The listing builds one solid part. Answer for the finished solid, in the listing's coordinates (mm). A direction names the side the tool comes from. Round coordinates to 2 decimals unless told otherwise and drop trailing zeros. Order: outer loops, then holes, each group sorted by start corner. A loop starts at its lowest first (then second) coordinate and runs counter-clockwise, first axis right, second up. Notation, with made-up numbers: (-2, 62.5) - (12, 62.5) arc R20 cw to (12, 90.5) - close; hole circle Ø7 at (57, 50). An arc over 180 degrees is marked (long way). Write item = value, one per line.
from build123d import *

# Parameters (mm, degrees)
SKETCH1_R                      = 27.505813168
SKETCH1_R_2                    = 25.505813168
BOSS_EXTRUDE1_DEPTH            = 30
SKETCH2_R                      = 27.505813168
SKETCH2_R_2                    = 25.505813168
BOSS_EXTRUDE4_DEPTH            = 6
SKETCH2_4_R                    = 25.505813168
SKETCH2_4_R_2                  = 10.5
BOSS_EXTRUDE5_DEPTH            = 4
SKETCH2_5_R                    = 10.5
BOSS_EXTRUDE6_DEPTH            = 2
SKETCH3_R                      = 27.505813168
SKETCH3_R_2                    = 25.505813168
SKETCH3_R_3                    = 21.505813168
SKETCH3_W                      = 4
SKETCH3_H                      = 13
BOSS_EXTRUDE8_DEPTH            = 6
CUT_EXTRUDE3_REACH             = 53.664
CUT_EXTRUDE4_REACH             = 55.001
SKETCH9_R                      = 1
CUT_EXTRUDE4_DIRECTION_2_DEPTH = 54.001316173
FILLET9_R                      = 10
FILLET10_R                     = 1


# Some blends are built 0.0001 mm under size
with BuildPart() as part:
    # Sketch1 → Boss-Extrude1 (new body)
    with BuildSketch(Plane.YZ):
        with Locations(Location((0, 0, 0), (0, 0, 270))):
            Circle(SKETCH1_R)
        with Locations(Location((0, 0, 0), (0, 0, 270))):
            Circle(SKETCH1_R_2, mode=Mode.SUBTRACT)
    extrude(amount=BOSS_EXTRUDE1_DEPTH)

    # Sketch2 → Boss-Extrude4 (add)
    with BuildSketch(Plane.YZ.offset(30)):
        with Locations(Location((0, 0, 0), (0, 0, 270))):
            Circle(SKETCH2_R)
        with Locations(Location((0, 0, 0), (0, 0, 270))):
            Circle(SKETCH2_R_2, mode=Mode.SUBTRACT)
    extrude(amount=BOSS_EXTRUDE4_DEPTH)

    # Sketch2<4> → Boss-Extrude5 (add)
    with BuildSketch(Plane.YZ.offset(30)):
        with Locations(Location((0, 0, 0), (0, 0, 270))):
            Circle(SKETCH2_4_R)
        with Locations(Location((0, 0, 0), (0, 0, 270))):
            Circle(SKETCH2_4_R_2, mode=Mode.SUBTRACT)
    extrude(amount=BOSS_EXTRUDE5_DEPTH)

    # Sketch2<5> → Boss-Extrude6 (add)
    with BuildSketch(Plane.YZ.offset(30)):
        with Locations(Location((0, 0, 0), (0, 0, 270))):
            Circle(SKETCH2_5_R)
    extrude(amount=BOSS_EXTRUDE6_DEPTH)

    # Sketch3 → Boss-Extrude8 (add)
    # profile 1 of 6: a face of its own
    with BuildSketch(Plane(origin=(0, 0, 0), x_dir=(0, -1, 0), z_dir=(-1, 0, 0))):
        with Locations(Location((0, 0, 0), (0, 0, 270))):
            Circle(SKETCH3_R)
        with Locations(Location((0, 0, 0), (0, 0, 270))):
            Circle(SKETCH3_R_2, mode=Mode.SUBTRACT)
    # profile 2 of 6: a face of its own
    with BuildSketch(Plane(origin=(0, 0, 0), x_dir=(0, -1, 0), z_dir=(-1, 0, 0))):
        with Locations(Location((0, 0, 0), (0, 0, 270))):
            Circle(SKETCH3_R_2)
        Circle(SKETCH3_R_3, mode=Mode.SUBTRACT)
    # profile 3 of 6: a face of its own
    with BuildSketch(Plane(origin=(0, 0, 0), x_dir=(0, -1, 0), z_dir=(-1, 0, 0))):
        with BuildLine():
            ThreePointArc((12.5, 0), (3.375390485, 12.035644523), (-10.677078252, 6.5))
            Line((-10.677078252, 6.5), (0, 6.5))
            Line((0, 6.5), (7.5, 6.5))
            Line((7.5, 6.5), (7.5, -6.5))
            Line((7.5, -6.5), (0, -6.5))
            Line((0, -6.5), (-10.677078252, -6.5))
            ThreePointArc((-10.677078252, -6.5), (3.375390485, -12.035644523), (12.5, 0))
        make_face()
    # profile 4 of 6: a face of its own
    with BuildSketch(Plane(origin=(0, 0, 0), x_dir=(0, -1, 0), z_dir=(-1, 0, 0))):
        with BuildLine():
            Line((-20.5, -6.5), (-20.5, 6.5))
            ThreePointArc((-20.5, 6.5), (-21.505813168, 0), (-20.5, -6.5))
        make_face()
    # profile 5 of 6: a face of its own
    with BuildSketch(Plane(origin=(0, 0, 0), x_dir=(0, -1, 0), z_dir=(-1, 0, 0))):
        with BuildLine():
            Line((-20.5, 6.5), (-16.5, 6.5))
            Line((-16.5, 6.5), (-10.677078252, 6.5))
            ThreePointArc((-10.677078252, 6.5), (3.375390485, 12.035644523), (12.5, 0))
            ThreePointArc((12.5, 0), (3.375390485, -12.035644523), (-10.677078252, -6.5))
            Line((-10.677078252, -6.5), (-16.5, -6.5))
            Line((-16.5, -6.5), (-20.5, -6.5))
            ThreePointArc((-20.5, -6.5), (3.288679831, -21.252872393), (21.505813168, 0))
            ThreePointArc((21.505813168, 0), (3.288679831, 21.252872393), (-20.5, 6.5))
        make_face()
    # profile 6 of 6: a face of its own
    with BuildSketch(Plane(origin=(0, 0, 0), x_dir=(0, -1, 0), z_dir=(-1, 0, 0))):
        with Locations((-18.5, 0)):
            Rectangle(SKETCH3_W, SKETCH3_H)
    extrude(amount=-BOSS_EXTRUDE8_DEPTH)

    # Sketch8 → Cut-Extrude3 (cut, up to next)
    with BuildSketch(Plane.YZ.offset(34), mode=Mode.PRIVATE) as cut_extrude3_sk1:
        with BuildLine():
            Line((-13.266499161, -2.5), (-22.360679775, -2.5))
            ThreePointArc((-22.360679775, -2.5), (-15.909902577, -15.909902577), (-2.5, -22.360679775))
            Line((-2.5, -22.360679775), (-2.5, -13.266499161))
            ThreePointArc((-2.5, -13.266499161), (-9.545941546, -9.545941546), (-13.266499161, -2.5))
        make_face()
    cut_extrude3_tool1 = extrude(cut_extrude3_sk1.sketch, amount=-CUT_EXTRUDE3_REACH, mode=Mode.PRIVATE) & part.part
    # Sketch8 → Cut-Extrude3 (cut, up to next)
    with BuildSketch(Plane.YZ.offset(34), mode=Mode.PRIVATE) as cut_extrude3_sk2:
        with BuildLine():
            Line((-2.5, 13.266499161), (-2.5, 22.360679775))
            ThreePointArc((-2.5, 22.360679775), (-15.909902577, 15.909902577), (-22.360679775, 2.5))
            Line((-22.360679775, 2.5), (-13.266499161, 2.5))
            ThreePointArc((-13.266499161, 2.5), (-9.545941546, 9.545941546), (-2.5, 13.266499161))
        make_face()
    cut_extrude3_tool2 = extrude(cut_extrude3_sk2.sketch, amount=-CUT_EXTRUDE3_REACH, mode=Mode.PRIVATE) & part.part
    # Sketch8 → Cut-Extrude3 (cut, up to next)
    with BuildSketch(Plane.YZ.offset(34), mode=Mode.PRIVATE) as cut_extrude3_sk3:
        with BuildLine():
            ThreePointArc((22.360679775, 2.5), (15.909902577, 15.909902577), (2.5, 22.360679775))
            Line((2.5, 22.360679775), (2.5, 13.266499161))
            ThreePointArc((2.5, 13.266499161), (9.545941546, 9.545941546), (13.266499161, 2.5))
            Line((13.266499161, 2.5), (22.360679775, 2.5))
        make_face()
    cut_extrude3_tool3 = extrude(cut_extrude3_sk3.sketch, amount=-CUT_EXTRUDE3_REACH, mode=Mode.PRIVATE) & part.part
    # Sketch8 → Cut-Extrude3 (cut, up to next)
    with BuildSketch(Plane.YZ.offset(34), mode=Mode.PRIVATE) as cut_extrude3_sk4:
        with BuildLine():
            ThreePointArc((2.5, -22.360679775), (15.909902577, -15.909902577), (22.360679775, -2.5))
            Line((22.360679775, -2.5), (13.266499161, -2.5))
            ThreePointArc((13.266499161, -2.5), (9.545941546, -9.545941546), (2.5, -13.266499161))
            Line((2.5, -13.266499161), (2.5, -22.360679775))
        make_face()
    cut_extrude3_tool4 = extrude(cut_extrude3_sk4.sketch, amount=-CUT_EXTRUDE3_REACH, mode=Mode.PRIVATE) & part.part
    add(cut_extrude3_tool1.solids().sort_by_distance((34, -12.15155, -12.15155))[0], mode=Mode.SUBTRACT)
    add(cut_extrude3_tool2.solids().sort_by_distance((34, -12.15155, 12.15155))[0], mode=Mode.SUBTRACT)
    add(cut_extrude3_tool3.solids().sort_by_distance((34, 12.15155, 12.15155))[0], mode=Mode.SUBTRACT)
    add(cut_extrude3_tool4.solids().sort_by_distance((34, 12.15155, -12.15155))[0], mode=Mode.SUBTRACT)

    # Sketch9 → Cut-Extrude4 (cut, up to next)
    with BuildSketch(Plane(origin=(0, 0, 0), x_dir=(0, -1, 0), z_dir=(-1, 0, 0)), mode=Mode.PRIVATE) as cut_extrude4_sk1:
        with Locations(Location((-10.5, 10.5, 0), (0, 0, 270))):
            Circle(SKETCH9_R)
    cut_extrude4_tool1 = extrude(cut_extrude4_sk1.sketch, amount=-CUT_EXTRUDE4_REACH, mode=Mode.PRIVATE) & part.part
    # Sketch9 → Cut-Extrude4 (cut, up to next)
    with BuildSketch(Plane(origin=(0, 0, 0), x_dir=(0, -1, 0), z_dir=(-1, 0, 0)), mode=Mode.PRIVATE) as cut_extrude4_sk2:
        with Locations(Location((10.5, 10.5, 0), (0, 0, 270))):
            Circle(SKETCH9_R)
    cut_extrude4_tool2 = extrude(cut_extrude4_sk2.sketch, amount=-CUT_EXTRUDE4_REACH, mode=Mode.PRIVATE) & part.part
    # Sketch9 → Cut-Extrude4 (cut, up to next)
    with BuildSketch(Plane(origin=(0, 0, 0), x_dir=(0, -1, 0), z_dir=(-1, 0, 0)), mode=Mode.PRIVATE) as cut_extrude4_sk3:
        with Locations(Location((10.5, -10.5, 0), (0, 0, 270))):
            Circle(SKETCH9_R)
    cut_extrude4_tool3 = extrude(cut_extrude4_sk3.sketch, amount=-CUT_EXTRUDE4_REACH, mode=Mode.PRIVATE) & part.part
    # Sketch9 → Cut-Extrude4 (cut, up to next)
    with BuildSketch(Plane(origin=(0, 0, 0), x_dir=(0, -1, 0), z_dir=(-1, 0, 0)), mode=Mode.PRIVATE) as cut_extrude4_sk4:
        with Locations(Location((-10.5, -10.5, 0), (0, 0, 270))):
            Circle(SKETCH9_R)
    cut_extrude4_tool4 = extrude(cut_extrude4_sk4.sketch, amount=-CUT_EXTRUDE4_REACH, mode=Mode.PRIVATE) & part.part
    add(cut_extrude4_tool1.solids().sort_by_distance((0, 10.5, 10.5))[0], mode=Mode.SUBTRACT)
    add(cut_extrude4_tool2.solids().sort_by_distance((0, -10.5, 10.5))[0], mode=Mode.SUBTRACT)
    add(cut_extrude4_tool3.solids().sort_by_distance((0, -10.5, -10.5))[0], mode=Mode.SUBTRACT)
    add(cut_extrude4_tool4.solids().sort_by_distance((0, 10.5, -10.5))[0], mode=Mode.SUBTRACT)

    # Sketch9 → Cut-Extrude4 direction 2 (cut)
    with BuildSketch(Plane(origin=(0, 0, 0), x_dir=(0, -1, 0), z_dir=(-1, 0, 0))):
        with Locations(Location((-10.5, 10.5, 0), (0, 0, 270))):
            Circle(SKETCH9_R)
        with Locations(Location((10.5, 10.5, 0), (0, 0, 270))):
            Circle(SKETCH9_R)
        with Locations(Location((10.5, -10.5, 0), (0, 0, 270))):
            Circle(SKETCH9_R)
        with Locations(Location((-10.5, -10.5, 0), (0, 0, 270))):
            Circle(SKETCH9_R)
    extrude(amount=CUT_EXTRUDE4_DIRECTION_2_DEPTH, mode=Mode.SUBTRACT)

    # Fillet9
    # the kernel refuses this fillet: 10 mm, written as the material it takes off along each edge
    with BuildSketch(Plane(origin=(0, 0, 0), x_dir=(0, 0, -1), z_dir=(0, -1, 0))) as fillet9_piece_1:
        with BuildLine():
            CenterArc((27.505813168 - FILLET9_R, FILLET9_R), FILLET9_R, 270, 90)
            Line((27.505813168 - FILLET9_R, 0), (27.505813168, 0))
            Line((27.505813168, 0), (27.505813168, FILLET9_R))
        make_face()
    revolve(axis=Axis((0, 0, 0), (1, 0, 0)), mode=Mode.SUBTRACT)

    # Fillet10
    fillet10_edges = [part.edges().sort_by_distance(p)[0] for p in [
        (36, 0, 27.505813168),
        (36, 0, 25.505813168),
    ]]
    fillet(fillet10_edges, radius=FILLET10_R - 0.0001)  # a hair under: the kernel refuses the full size


solid = part.part
Q1. Find the intervals of material crossed by line 1 (X direction, y = 2, z = -13.5); line 2 (Z direction, x = 3.6, y = 10.5); line 3 (Y direction, x = 33, z = 0), in increasing order. Write a range as from..to.
Model answer:
line_1 = 0..6, 30..34
line_2 = -22.9..-11.5, -9.5..-6.5, 6.5..9.5, 11.5..22.9
line_3 = -27.51..-10.5, 10.5..27.51
Q2. Section C-C on x = 12 is taken. Determine the outline of the cut face in (y, z).
Model answer:
outline = circle Ø55.01 at (0, 0); hole circle Ø51.01 at (0, 0)
Q3. For faces 1 (the face through (6, -11, 0)), 2 (the face through (2.96, -11.49, 10.63)), 3 (the face through (3, 4, -6.5)), 4 (the face through (32, -2.5, -18)), determine the directions among +Z, -Z, +X, -X, +Y, -Y from which every point of the face is accessible in a straight line to the end or side of a thin tool.
Model answer:
face_1 = none
face_2 = +X, -X
face_3 = -X
face_4 = +X
Q4. Flat-ended cylindrical pins translate along their axes: P1, Ø10, axis at x = 14.5, z = 10.5, coming from the +Y side; P2, Ø12, axis at x = 10.5, y = -8, coming from the -Z side; P3, Ø5, axis at x = 3, z = -2, coming from the +Y side. Find the tip coordinate at first contact, or state that the pin passes through.
Model answer:
P1 = 26.95
P2 = -27.43
P3 = 26.37
Q5. Section D-D on y = -6 is taken. Count the separate pieces of the cut face and the enclosed holes in it, then the cut area to 3 significant figures.
Model answer:
separate_pieces = 3
enclosed_holes = 0
area = 409 mm^2
